Geometry: see drawing. Coordinates: mm, zero at the bounding-box minimum. A direction names the side the tool comes from. Give positions to 0.01 mm unless a question says otherwise; leave off trailing zeros. Write each loop counter-clockwise with the first axis right and the second up, starting at its lowest first coordinate (ties: lowest second). Pieces come first, ordered by that corner, then holes. Notation, with made-up numbers: M -28.75,-9 L -9.75,-9 A20 ccw -9.75,14 Z; hole C 50,-31.75 d9. An arc over 180 degrees is marked long. Use a Markdown table: item, result. Add a question column.
(1) Cut plane A-A (y = 2.75). Output: boundary loops of the cut face in (x, z).
(2) Cut plane B-B (z = 4). Output: boundary loops of the cut face in (x, y).
(3) Reachability of the marked faces 1 and 2 from +Z, -Z, +X, -X, +Y, -Y: full face, straight path, thin tool, end or side. Return the list, or none.
(4) Cut plane C-C (y = 1.75). Output: boundary loops of the cut face in (x, z).
(5) Material intervals for L1, parallel to Z at x = 2.15, y = 1; L2, parallel to Z at x = 3.05, y = 3.6; L3, parallel to Y at x = 1.95, z = 13, sorted ascending.
(6) Pin query (flat end, axial travel): pin 1 Ø0.7 at (y, z) = (2.5, 26) entering from +X; pin 2 Ø1 at (x, y) = (2.5, 2.5) entering from +Z; pin 3 Ø1.5 at (x, z) = (1, 17.5) entering from +Y; pin 4 Ø2 at (x, z) = (3.5, 19.5) entering from +Y. Return the tip coordinate at first contact, or that it passes through.
(7) Cut plane D-D (z = 25). Output: boundary loops of the cut face in (x, y).
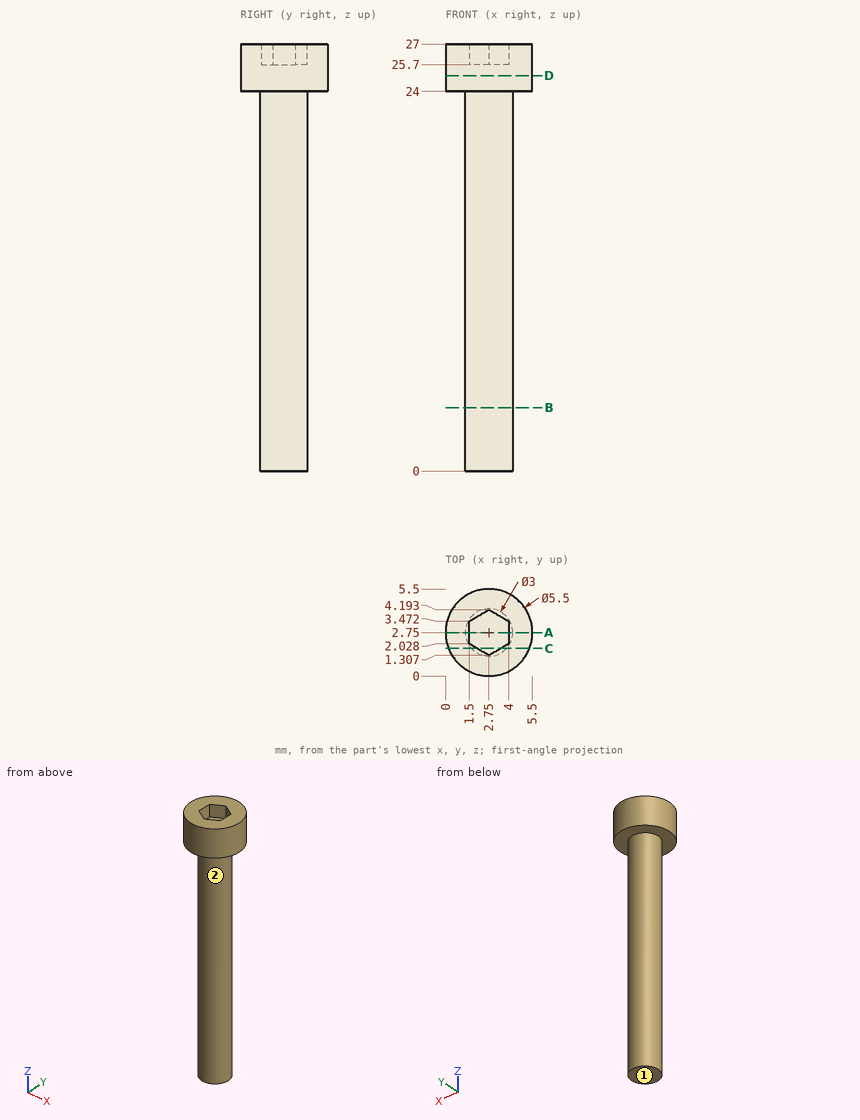
Answer list:
| question | item | result |
|---|---|---|
| 1 | outline | M 0,24 L 1.25,24 L 1.25,0 L 4.25,0 L 4.25,24 L 5.5,24 L 5.5,27 L 4,27 L 4,25.7 L 1.5,25.7 L 1.5,27 L 0,27 Z |
| 2 | outline | C 2.75,2.75 d3 |
| 3 | face 1 | -Z, +X, -X, +Y, -Y |
| 3 | face 2 | -Z |
| 4 | outline | M 0.19,24 L 1.63,24 L 1.63,0 L 3.87,0 L 3.87,24 L 5.31,24 L 5.31,27 L 3.52,27 L 3.52,25.7 L 1.98,25.7 L 1.98,27 L 0.19,27 Z |
| 5 | L1 | 24 to 27 |
| 5 | L2 | 0 to 25.7 |
| 5 | L3 | 1.48 to 4.02 |
| 6 | pin 1 | x = 5.5 |
| 6 | pin 2 | z = 25.7 |
| 6 | pin 3 | y = 3.87 |
| 6 | pin 4 | y = 4.25 |
| 7 | outline | C 2.75,2.75 d5.5 |
